The figure shows three views and two pictorial views of one solid part (mm, origin at its lowest corner). Answer the questions. A direction names the side the tool comes from. Give positions to 0.01 mm unless a question says otherwise; leave off trailing zeros. Write each loop counter-clockwise with the first axis right and the second up, starting at its lowest first coordinate (ties: lowest second). Pieces come first, ordered by that corner, then holes. Notation, with made-up numbers: M 49.5,-30.5 L 104.5,-30.5 A24 cw 104.5,-19.5 Z; hole C 56.5,-30 d8. An arc over 180 degrees is marked long. Return JSON: item names as keys, results as strings.
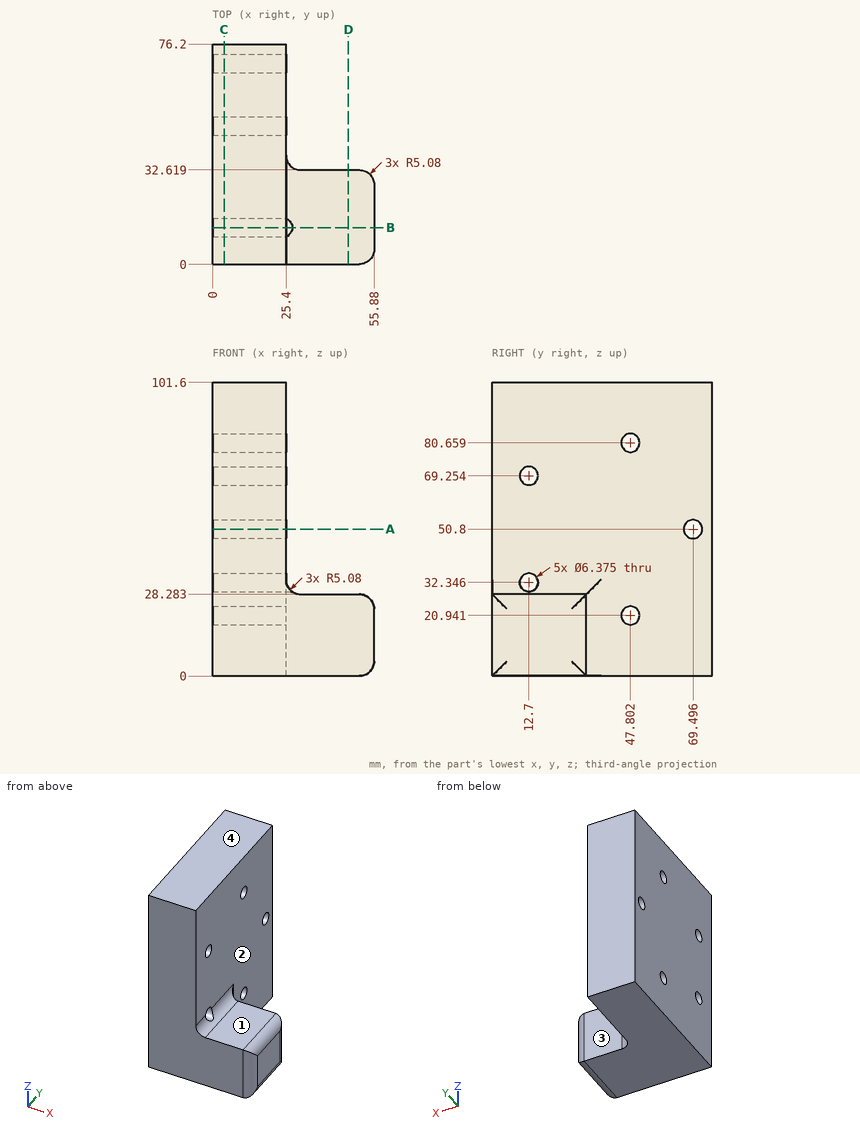
Item 1: A cutting plane is placed at B-B, the plane y = 12.7. Write down the section's boundary in (x, z).
Geometry results:
{"outline": "M 0,0 L 50.8,0 A5.08 ccw 55.88,5.08 L 55.88,23.2 A5.08 ccw 50.8,28.28 L 30.48,28.28 A5.08 cw 27.63,29.16 L 0,29.16 Z; M 0,35.53 L 25.4,35.53 L 25.4,66.07 L 0,66.07 Z; M 0,72.44 L 25.4,72.44 L 25.4,101.6 L 0,101.6 Z"}
Item 2: Which of the six approach directions +Z, -Z, +X, -X, +Y, -Y give full straight-line access (tool end or side, diameter ignored) to the marked faces 1, 2, 3 and 4?
Geometry results:
{"face 1": "+Z, +X, +Y, -Y", "face 2": "+Z, +X, +Y", "face 3": "+Z, -Z, +X, +Y", "face 4": "+Z, +X, -X, +Y, -Y"}
Item 3: A cutting plane is placed at A-A, the plane z = 50.8. Write down the section's boundary in (x, y).
Geometry results:
{"outline": "M 0,0 L 25.4,0 L 25.4,66.31 L 0,66.31 Z; M 0,72.68 L 25.4,72.68 L 25.4,76.2 L 0,76.2 Z"}
Item 4: Given pin 1 Ø10 at (y, z) = (47.8, 20.94) entering from +X; pin 2 Ø6 at (x, y) = (36.5, 17.5) entering from +Z; pin 3 Ø22.5 at (x, z) = (44, 17) entering from +Y, each flat-ended and moving along its own axis, determine where each tip first touches the part or whether it passes through.
Geometry results:
{"pin 1": "stops at x = 25.4", "pin 2": "stops at z = 28.28", "pin 3": "stops at y = 32.62"}
Item 5: A cutting plane is placed at D-D, the plane x = 47. Write down the section's boundary in (y, z).
Geometry results:
{"outline": "M 0,0 L 32.62,0 L 32.62,28.28 L 0,28.28 Z"}
Item 6: Find the intervals of material crossed by line 1 (Z direction, x = 17.5, y = 12.7); line 2 (Y direction, x = 51, z = 17) (1 decimal); line 3 (X direction, y = 48, z = 95.5), in increasing order.
Geometry results:
{"line 1": "z = 0 to 29.16, 35.53 to 66.07, 72.44 to 101.6", "line 2": "y = 0 to 32.6", "line 3": "x = 0 to 25.4"}
Item 7: A cutting plane is placed at C-C, the plane x = 4. Write down the section's boundary in (y, z) (1 decimal).
Geometry results:
{"outline": "M 0,0 L 76.2,0 L 76.2,101.6 L 0,101.6 Z; hole C 12.7,32.3 d6.4; hole C 12.7,69.3 d6.4; hole C 47.8,20.9 d6.4; hole C 47.8,80.7 d6.4; hole C 69.5,50.8 d6.4"}
